Can you work these out from the drawing? Everything is in mm from the part's minimum corner. A direction names the side the tool comes from. Give positions to 0.01 mm unless a question says otherwise; leave off trailing zeros. Loops run counter-clockwise (first coordinate to the right, second up) from the corner with the lowest first, then second, coordinate; pieces in that order, holes last. Notation, with made-up numbers: (-15, 68) -> (-9, 68) arc R8 ccw to (-9, 80) -> close; hole circle Ø7 at (55, -15.5). An arc over 180 degrees is marked (long way). Write item = value, one per line. Start each with the question number.
1) On a 3-axis mill with a long thin cutter (end or side, diameter ignored), from which of +Z, -Z, +X, -X, +Y, -Y can I reach the whole of each face in a straight line? I mean the marked faces 5 and 6. Say none if no direction works.
2) I'm going to push flat-ended pins straight in: pin 1 Ø7 at (x, z) = (28.5, 28.5) entering from -Y; pin 2 Ø12 at (y, z) = (5.5, 43.5) entering from +X; pin 3 Ø1.5 at (y, z) = (6, 25.5) entering from +X; pin 4 Ø3 at (y, z) = (2.5, 39.5) entering from +X. Where does each tip first touch, or does it pass through?
3) I want a section at A-A (x = 5). List the corners of the cut face in (y, z) for me (1 decimal).
4) I want a section at C-C (x = 38.5). List the corners of the cut face in (y, z) for me.
5) I need wall thicknesses on probe 1 along Y at (x, z) = (28.5, 39); probe 2 along Z at (x, y) = (42.5, 2) (1 decimal); probe 3 along Y at (x, z) = (42, 52). Which ranges of each line are inside material? Lowest first, please. Write a range as from..to.
6) I want a section at B-B (z = 23.5). List the corners of the cut face in (x, y) for me.
7) I want a section at D-D (y = 23.75). List the corners of the cut face in (x, z) for me, and give its area (3 significant figures).
8) If we mould it in two halves opening along X, with no side actions, what happens to the marked faces 1, 2, 3 and 4? For each: +X half, -X half, draft (parallel to the pull), parting line (faces both ways), or undercut.
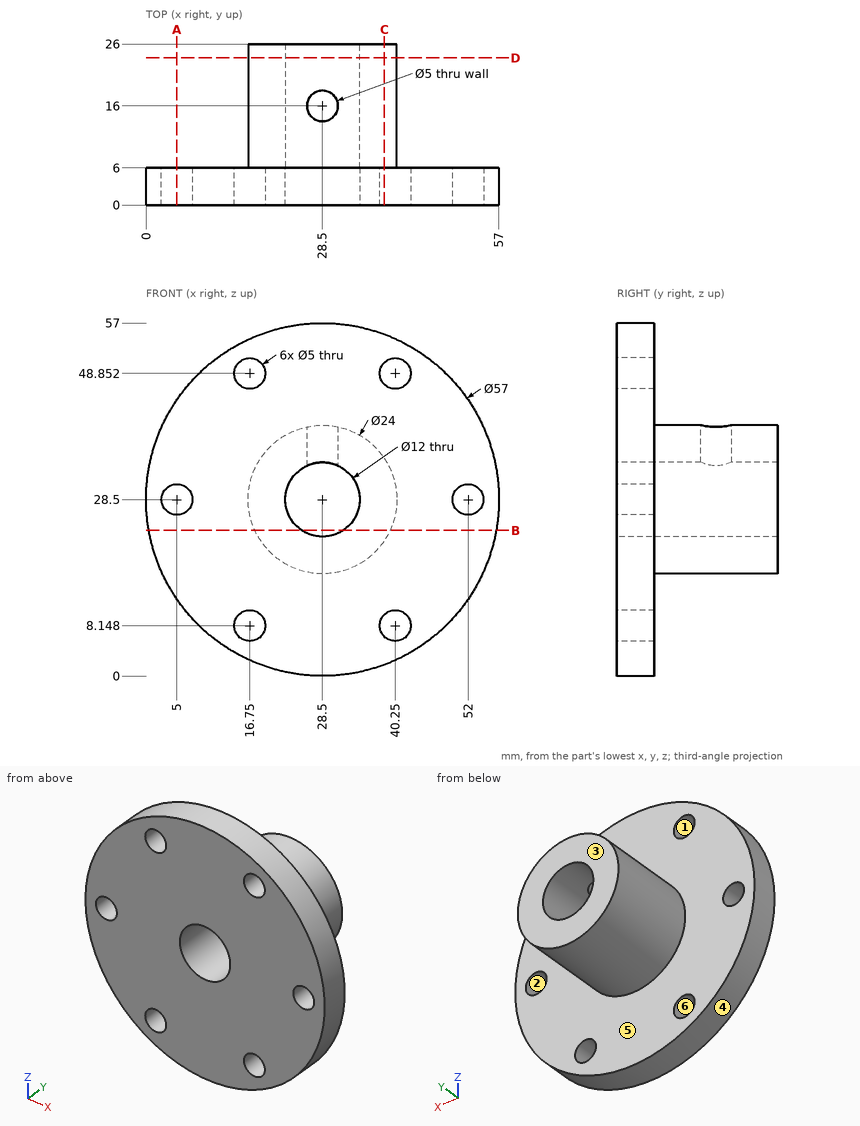
Answer list:
q1.face_5 = +Y
q1.face_6 = +Y, -Y
q2.pin_1 = through
q2.pin_2 = 55.54
q2.pin_3 = 56.91
q2.pin_4 = 55.37
q3.outline = (0, 12.4) -> (6, 12.4) -> (6, 26) -> (0, 26) -> close; (0, 31) -> (6, 31) -> (6, 44.6) -> (0, 44.6) -> close
q4.outline = (0, 1.81) -> (6, 1.81) -> (6, 6.36) -> (0, 6.36) -> close; (0, 9.93) -> (6, 9.93) -> (6, 21.87) -> (26, 21.87) -> (26, 35.13) -> (6, 35.13) -> (6, 47.07) -> (0, 47.07) -> close; (0, 50.64) -> (6, 50.64) -> (6, 55.19) -> (0, 55.19) -> close
q5.probe_1 = 0..13.5, 18.5..26
q5.probe_2 = 3.7..7.1, 9.2..47.8, 49.9..53.3
q5.probe_3 = 0..6
q6.outline = (0.44, 0) -> (25.18, 0) -> (25.18, 26) -> (17.59, 26) -> (17.59, 6) -> (0.44, 6) -> close; (31.82, 0) -> (56.56, 0) -> (56.56, 6) -> (39.41, 6) -> (39.41, 26) -> (31.82, 26) -> close
q7.outline = circle Ø24 at (28.5, 28.5); hole circle Ø12 at (28.5, 28.5)
q7.area = 339 mm^2
q8.face_1 = undercut
q8.face_2 = undercut
q8.face_3 = draft
q8.face_4 = parting line
